Build history of the part. All positions in model axes, mm. A direction names the side the tool comes from. Coordinates: 2 decimals unless noted, no trailing zeros. Order: outer loops, then holes, each group sorted by start corner. A loop starts at its lowest first (then second) coordinate and runs counter-clockwise, first axis right, second up. Notation, with made-up numbers: (-22, 87.25) - (28, 87.25) arc R18 ccw to (28, 110.25) - close; hole circle Ø8 at (-30.75, -12). An arc over 180 degrees is marked (long way). Write each question's results on one line, items separated by ' | '.
from build123d import *

# Parameters (mm, degrees)
SKETCH1_R                = 21.209
BOSS_EXTRUDE1_DEPTH      = 50.8
CUT_EXTRUDE2_DEPTH       = 59.993926484
BOSS_EXTRUDE3_REACH      = 111.794
BOSS_EXTRUDE3_END_RADIUS = 21.209
BOSS_EXTRUDE3_START      = -50.8
SKETCH4_W                = 101.6
SKETCH4_H                = 42.418
CUT_EXTRUDE1_DEPTH       = 75.907287332
CUT_EXTRUDE1_DEPTH_BACK  = 75.907287332
SKETCH2_R                = 12.7
SKETCH5_W                = 101.6
SKETCH5_H                = 88.9
BOSS_EXTRUDE4_DEPTH      = 3.175


with BuildPart() as part:
    # Sketch1 → Boss-Extrude1 (new, symmetric)
    with BuildSketch(Plane(origin=(0, 0, 0), x_dir=(0, 0, -1), z_dir=(1, 0, 0))):
        Circle(SKETCH1_R)
        with BuildLine():
            Line((15.617902132, -9.017), (7.366, -8.295052111))
            Line((7.366, -8.295052111), (7.366, 9.017))
            Line((7.366, 9.017), (15.617902132, 9.017))
            ThreePointArc((15.617902132, 9.017), (-18.034, 0), (15.617902132, -9.017))
        make_face(mode=Mode.SUBTRACT)
    extrude(amount=BOSS_EXTRUDE1_DEPTH, both=True)

    # Sketch3 → Cut-Extrude2 (cut, through all)
    with BuildSketch(Plane(origin=(0, 0, 0), x_dir=(1, 0, 0), z_dir=(0, 1, 0))):
        with BuildLine():
            Line((-12.7, -6.35), (-12.7, -32.196981008))
            Line((-12.7, -32.196981008), (12.7, -32.196981008))
            Line((12.7, -32.196981008), (12.7, -6.35))
            ThreePointArc((12.7, -6.35), (0, 6.35), (-12.7, -6.35))
        make_face()
    extrude(amount=CUT_EXTRUDE2_DEPTH, mode=Mode.SUBTRACT)

    # Boss-Extrude3: up to this cylinder (the profile starts outside it)
    boss_extrude3_end = Plane(origin=(0, 0, 0), z_dir=(-1, 0, 0)) * Cylinder(BOSS_EXTRUDE3_END_RADIUS, 267.006, mode=Mode.PRIVATE)
    # Sketch4 → Boss-Extrude3 (add, up to the surface)
    with BuildSketch(Plane(origin=(0, 0, 0), x_dir=(1, 0, 0), z_dir=(0, 1, 0)).offset(BOSS_EXTRUDE3_START), mode=Mode.PRIVATE) as boss_extrude3_sk1:
        Rectangle(SKETCH4_W, SKETCH4_H)
    boss_extrude3_tool1 = extrude(boss_extrude3_sk1.sketch, amount=BOSS_EXTRUDE3_REACH, mode=Mode.PRIVATE) - boss_extrude3_end
    add(boss_extrude3_tool1.solids().sort_by_distance((0, -50.8, 0))[0])

    # Sketch2 → Cut-Extrude1 (cut, two sides: drawn at the far end of the back side and taken through both)
    with BuildSketch(Plane.XY.offset(-CUT_EXTRUDE1_DEPTH_BACK)):
        Circle(SKETCH2_R)
    extrude(amount=CUT_EXTRUDE1_DEPTH + CUT_EXTRUDE1_DEPTH_BACK, mode=Mode.SUBTRACT)

    # Sketch5 → Boss-Extrude4 (add)
    with BuildSketch(Plane.XZ.offset(50.8)):
        Rectangle(SKETCH5_W, SKETCH5_H)
        with BuildLine():
            Line((44.45, 41.275), (-44.45, 41.275))
            ThreePointArc((-44.45, 41.275), (-47.625, 38.1), (-44.45, 34.925))
            Line((-44.45, 34.925), (44.45, 34.925))
            ThreePointArc((44.45, 34.925), (47.625, 38.1), (44.45, 41.275))
        make_face(mode=Mode.SUBTRACT)
        with BuildLine():
            Line((44.45, -41.275), (-44.45, -41.275))
            ThreePointArc((-44.45, -41.275), (-47.625, -38.1), (-44.45, -34.925))
            Line((-44.45, -34.925), (44.45, -34.925))
            ThreePointArc((44.45, -34.925), (47.625, -38.1), (44.45, -41.275))
        make_face(mode=Mode.SUBTRACT)
    extrude(amount=-BOSS_EXTRUDE4_DEPTH)


solid = part.part
1. Drop flat-ended pins along their axis: pin 1 Ø4 at (x, z) = (-30.5, -11) entering from +Y; pin 2 Ø7 at (x, z) = (-21, 37.5) entering from +Y (3 decimals); pin 3 Ø3 at (x, y) = (-28.5, -27) entering from -Z; pin 4 Ø6 at (x, y) = (-8.5, -1.5) entering from +Z. Give the stop position or say it passes through.
Solved:
pin 1: stops at y = 19.2 | pin 2: stops at y = -47.625 | pin 3: stops at z = -21.21 | pin 4: passes through
2. Band-saw the part on B-B on z = -38.1. Give the cut face in (x, y) (3 decimals), then the cut area to 3 significant figures.
Solved:
outline: (-50.8, -50.8) - (-47.625, -50.8) - (-47.625, -47.625) - (-50.8, -47.625) - close; (47.625, -50.8) - (50.8, -50.8) - (50.8, -47.625) - (47.625, -47.625) - close | area: 20.2 mm2
3. Tool access for faces 1 (the face through (30, 9.017, -11)), 2 (the face through (-1, -47.625, -30)), 3 (the face through (1, -49, -41.275)), 4 (the face through (-1, -47.625, 30)): list every direction of +Z, -Z, +X, -X, +Y, -Y with a clear straight run to the whole face (end or side of a thin tool).
Solved:
face 1: +X, -X | face 2: -Z, +X, -X, +Y | face 3: +Y, -Y | face 4: +Z, +X, -X, +Y
4. Two-plate mould, pull along Z, no slides. Class faces 5 (the face through (-12.7, 11, 15)), 6 (the face through (-1, -49, -44.45)), 7 (the face through (-47.624, -49.235, 38.17)): +Z half, -Z half, draft (parallel to the pull), parting line (faces both ways), or undercut.
Solved:
face 5: draft | face 6: -Z half | face 7: undercut
5. Band-saw the part on A-A on x = -28.5. Give the cut face in (y, z) (3 decimals), then the cut area to 3 significant figures.
Solved:
outline: (-50.8, -44.45) - (-47.625, -44.45) - (-47.625, -41.275) - (-50.8, -41.275) - close; (-50.8, -34.925) - (-47.625, -34.925) - (-47.625, -21.209) - (0, -21.209) arc R21.209 ccw to (0, 21.209) - (-47.625, 21.209) - (-47.625, 34.925) - (-50.8, 34.925) - close; (-50.8, 41.275) - (-47.625, 41.275) - (-47.625, 44.45) - (-50.8, 44.45) - close; hole (-9.017, -15.618) - (-8.295, -7.366) - (9.017, -7.366) - (9.017, -15.618) arc R18.034 ccw (long way) to start | area: 2,120 mm2
6. Band-saw the part on D-D on z = 0. Give the cut face in (x, y), then the cut area to 3 significant figures.
Solved:
outline: (-50.8, -50.8) - (50.8, -50.8) - (50.8, -18.03) - (-50.8, -18.03) - close; (-50.8, 18.03) - (-11, 18.03) - (-11, 21.21) - (-50.8, 21.21) - close; (11, 18.03) - (50.8, 18.03) - (50.8, 21.21) - (11, 21.21) - close | area: 3,580 mm2
7. Band-saw the part on C-C on x = 3.5. Give the cut face in (y, z) (3 decimals), then the cut area to 3 significant figures.
Solved:
outline: (-50.8, -44.45) - (-47.625, -44.45) - (-47.625, -41.275) - (-50.8, -41.275) - close; (-50.8, -34.925) - (-47.625, -34.925) - (-47.625, -21.209) - (-12.208, -21.209) - (-12.208, -13.273) arc R18.034 cw to (-12.208, 13.273) - (-12.208, 21.209) - (-47.625, 21.209) - (-47.625, 34.925) - (-50.8, 34.925) - close; (-50.8, 41.275) - (-47.625, 41.275) - (-47.625, 44.45) - (-50.8, 44.45) - close; (12.208, -17.343) arc R21.209 ccw to (20.384, -5.858) - (17.056, -5.858) arc R18.034 cw to (12.208, -13.273) - close | area: 1,670 mm2
8. Probe line 1 (Y direction, x = 18.5, z = 0); line 2 (X direction, y = 0, z = -16.75); line 3 (Y direction, x = 10, z = -14.5). List the from-to ranges inside material, lowest first.
Solved:
line 1: y = -50.8 to -18.03, 18.03 to 21.21 | line 2: x = -50.8 to -12.7, 12.7 to 50.8 | line 3: y = -50.8 to -10.72, -8.92 to -7.83, 7.83 to 9.02, 10.72 to 15.48
